Work out the finished part from the listing and answer in its coordinate system (mm). A direction names the side the tool comes from. Coordinates: 2 decimals unless noted, no trailing zeros. Order: outer loops, then holes, each group sorted by start corner. A loop starts at its lowest first (then second) coordinate and runs counter-clockwise, first axis right, second up. Notation, with made-up numbers: M 43.25,75.25 L 97.25,75.25 A20 ccw 97.25,112.25 Z; hole C 18.5,42 d5. An arc over 180 degrees is marked long. Write item = value, one per line. Start each with the question number.
Q1. Find section B-B on z = -28. Give the vertices of the cut face in (x, y).
Q2. Each of these flat-tipped pins is pushed along its axis until it touches: P1, Ø12, axis at y = 13, z = -5.5, coming from the +X side; P2, Ø3, axis at x = -5.5, z = 14, coming from the -Y side; P3, Ø12, axis at y = -3.5, z = 13, coming from the -X side. Where does it stop, or does it pass through?
Q3. Find section A-A on x = 20. Give the vertices of the cut face in (y, z).
Q4. Find section D-D on x = 0. Give the number of separate pieces and of enclosed holes in the cut face, and give its area (3 significant figures).
Q5. Find section C-C on y = 6. Give the vertices of the cut face in (x, z), and give its area (3 significant figures).
Q6. A tool of negligible diameter and unlimited length cuts with its end or side. For faces 1 (the cylindrical face through (23.846, 7.509, 37.465)), 2 (the cylindrical face through (-3.252, -14.643, 27.605)), 3 (the flat face through (-0.1, 13.4, -20)), from which of +Z, -Z, +X, -X, +Y, -Y can it reach the whole face along a straight path? Write none if from no direction.
Q7. Straight lines are drawn through the part: line 1 along Z through (x, y) = (-14, 1); line 2 along Y through (x, z) = (0, 37.9); line 3 along Y through (x, z) = (20, 36). For each, find the intervals that lie inside material, in ascending order.
Q8. Determine the mould class of faces 4 (the flat face through (3, -10, -35)), 5 (the cylindrical face through (-18.314, -0.221, 37.535)), 6 (the cylindrical face through (-3.252, -14.643, -27.395)) for opening direction X: released by +X, released by -X, zero draft, split by the parting line, or undercut.
```python
from build123d import *

# Parameters (mm, degrees)
SKETCH1_R           = 15
SKETCH1_R_2         = 10
BOSS_EXTRUDE1_DEPTH = 35
SKETCH5_W           = 3.556
SKETCH5_H           = 2.046
SKETCH6_R           = 25
SKETCH6_R_2         = 10
BOSS_EXTRUDE2_DEPTH = 5
CIRPATTERN1_COUNT   = 4


with BuildPart() as part:
    # Sketch1 → Boss-Extrude1 (new body, symmetric)
    with BuildSketch(Plane.XY):
        Circle(SKETCH1_R)
        Circle(SKETCH1_R_2, mode=Mode.SUBTRACT)
    extrude(amount=BOSS_EXTRUDE1_DEPTH, both=True)

    # Sketch5 → Cut-Revolve1 (revolve, cut)
    with BuildSketch(Plane(origin=(0, 0, 0), x_dir=(0, 0, -1), z_dir=(1, 0, 0))):
        with Locations((-18.222, 13.977)):
            Rectangle(SKETCH5_W, SKETCH5_H)
    cut_revolve1 = revolve(axis=Axis((0, 0, 0), (0, 0, 1)), mode=Mode.SUBTRACT)

    # Mirror1: Cut-Revolve1 across plane
    add(cut_revolve1.mirror(Plane.XY), mode=Mode.SUBTRACT)

    # Sketch6 → Boss-Extrude2 (add)
    with BuildSketch(Plane.XY.offset(35)):
        Circle(SKETCH6_R)
        Circle(SKETCH6_R_2, mode=Mode.SUBTRACT)
    extrude(amount=BOSS_EXTRUDE2_DEPTH)

    # Sketch9 → M3 Clearance Hole1 (revolve, cut)
    with BuildSketch(Plane(origin=(20, 0, 40), x_dir=(0, -1, 0), z_dir=(1, 0, 0))):
        Polygon((0, 0), (0, 18.521463052), (1.7, 17.5), (1.7, 0), align=None)
    m3_clearance_hole1 = revolve(axis=Axis((20, 0, 46.35), (0, 0, -1)), mode=Mode.SUBTRACT)

    # CirPattern1: M3 Clearance Hole1 ×4 about axis
    cirpattern1_axis = Axis((0, 0, 0), (0, 0, 1))
    for i in range(1, CIRPATTERN1_COUNT):
        add(m3_clearance_hole1.rotate(cirpattern1_axis, i * 360 / CIRPATTERN1_COUNT), mode=Mode.SUBTRACT)


solid = part.part
```
Findings below:
q1.outline = C 0,0 d30; hole C 0,0 d20
q2.P1 = 13.27
q2.P2 = -14.46
q2.P3 = -15
q3.outline = M -15,35 L -1.7,35 L -1.7,40 L -15,40 Z; M 1.7,35 L 15,35 L 15,40 L 1.7,40 Z
q4.separate_pieces = 4
q4.enclosed_holes = 0
q4.area = 787 mm^2
q5.outline = M -24.27,35 L -13.75,35 L -13.75,20 L -11.48,20 L -11.48,16.44 L -13.75,16.44 L -13.75,-16.44 L -11.48,-16.44 L -11.48,-20 L -13.75,-20 L -13.75,-35 L -8,-35 L -8,40 L -24.27,40 Z; M 8,-35 L 13.75,-35 L 13.75,-20 L 11.48,-20 L 11.48,-16.44 L 13.75,-16.44 L 13.75,16.44 L 11.48,16.44 L 11.48,20 L 13.75,20 L 13.75,35 L 24.27,35 L 24.27,40 L 8,40 Z
q5.area = 935 mm^2
q6.face_1 = +Z, -Z
q6.face_2 = -Z
q6.face_3 = none
q7.line_1 = -35 to -20, -16.44 to 16.44, 20 to 40
q7.line_2 = -25 to -21.7, -18.3 to -10, 10 to 18.3, 21.7 to 25
q7.line_3 = -15 to -1.7, 1.7 to 15
q8.face_4 = zero draft
q8.face_5 = undercut
q8.face_6 = split by the parting line
